from build123d import *

# Parameters (mm, degrees)
F0_W     = 3.6
F0_H     = 1.6955656027
F0_H_2   = 2
F1_DEPTH = 7


with BuildPart() as f1:
    # F0 (on Right) → F1 (new body)
    with BuildSketch(Plane.YZ):
        with Locations((-0.3402145463, -3.3855575087)):
            Rectangle(F0_W, F0_H)
        with Locations((-0.3402145463, -5.2333403101)):
            Rectangle(F0_W, F0_H_2)
        Polygon((-2.1402145463, -6.2333403101), (-2.1402145463, -4.2333403101), (-3.6402145463, -6.2333403101), align=None)
        Polygon((-3.3397897729, -2.5377747074), (-2.1402145463, -2.5377747074), (1.4597854537, -2.5377747074), (2.6593606802, -2.5377747074), (2.6593606802, -0.4877204478), (1.1097854537, -0.4877204478), (-0.3402145463, -0.4877204478), (-1.7902145463, -0.4877204478), (-3.3397897729, -0.4877204478), align=None)
        Polygon((2.9597854537, -6.2333403101), (1.4597854537, -4.2333403101), (1.4597854537, -6.2333403101), align=None)
        Polygon((-3.3402145463, -2.5377747074), (-3.3397897729, -2.5377747074), (-3.3397897729, -0.4877204478), (-4.7602145463, -0.4877204478), (-4.7602145463, 2.0122795522), (-4.508031692, 2.0122795522), (-4.7602145463, 3.5118722885), (-6.076728541, 3.5118722885), (-6.076728541, -2.5377747074), align=None)
        Polygon((2.6593606802, -0.4877204478), (2.6593606802, -2.5377747074), (2.6597854537, -2.5377747074), (5.3962994483, -2.5377747074), (5.3962994483, 3.5118722885), (4.0797854537, 3.5118722885), (3.8276025993, 2.0122795522), (4.0797854537, 2.0122795522), (4.0797854537, -0.4877204478), align=None)
        Polygon((-1.7902145463, 0.3914704144), (-1.7902145463, -0.4877204478), (-0.3402145463, -0.4877204478), (1.1097854537, -0.4877204478), (1.1097854537, 0.3914704144), (-0.3402145463, 0.3914704144), align=None)
    extrude(amount=F1_DEPTH)


solid = f1.part
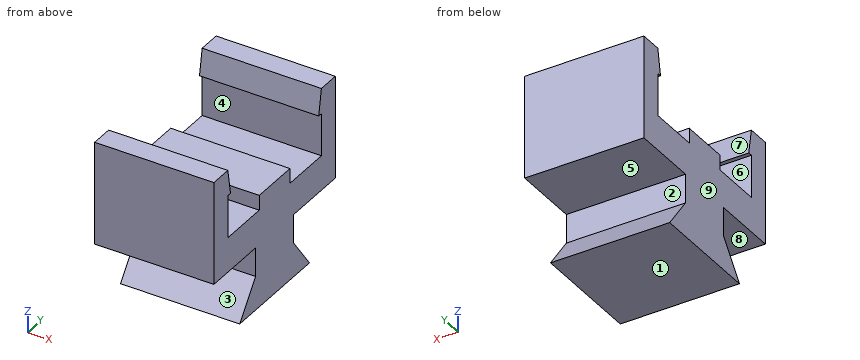
Check sheet for the modelled part. Datum: model origin and axes. Units: mm. Face numbers are marked on the shaded views. A direction names the side the tool comes from. Round coordinates to 2 decimals unless told otherwise and drop trailing zeros. Loops run counter-clockwise (first coordinate to the right, second up) from the corner with the lowest first, then second, coordinate; pieces in that order, holes last.
1. Sectioned sample at B-B on y = 2.5. Record the boundary of the cut face in (x, z).
2. Set-up check for the marked faces 5, 6, 7, 8 and 9: record each of +Z, -Z, +X, -X, +Y, -Y from which the full face is reachable in a straight line by a thin tool's end or side.
3. Mould release check, pull along Y, two halves, no side actions. Record for the marked faces 1, 2, 3 and 4: released by +Y, released by -Y, zero draft, split by the parting line, or undercut.
4. Sectioned sample at C-C on x = 6.75. Record the boundary of the cut face in (y, z), and give its area (3 significant figures).
5. Sectioned sample at D-D on z = -3.25. Record the boundary of the cut face in (x, y).
6. Scan lines: probe 1 along Y at (x, z) = (4.25, 0); probe 2 along Y at (x, z) = (6.25, 1.25); probe 3 along Y at (x, z) = (5.5, -3.5). Record each from-to range of solid material in increasing order.
7. Gauge pin test, flat ends, axial feed: pin 1 Ø1.2 at (x, y) = (4, 4.5) entering from -Z; pin 2 Ø0.5 at (x, z) = (3.5, -3.5) entering from +Y; pin 3 Ø1.5 at (x, y) = (2, 0) entering from +Z. Record the tip position at first contact, or that the pin passes through.
8. Sectioned sample at A-A on z = 2.75. Record the boundary of the cut face in (x, y).
Recorded:
1. outline: (0, -6.23) - (7, -6.23) - (7, -5.62) - (0, -5.62) - close; (0, -2.54) - (7, -2.54) - (7, -0.49) - (0, -0.49) - close
2. face 5: +X, -X, +Y
2. face 6: +X, -X
2. face 7: +Z, +X, -X
2. face 8: +X, -X, -Y
2. face 9: +Z, -Z, -X, +Y, -Y
3. face 1: zero draft
3. face 2: released by +Y
3. face 3: released by -Y
3. face 4: undercut
4. outline: (-6.08, -2.54) - (-2.14, -2.54) - (-2.14, -4.23) - (-3.64, -6.23) - (2.96, -6.23) - (1.46, -4.23) - (1.46, -2.54) - (5.4, -2.54) - (5.4, 3.51) - (4.08, 3.51) - (3.83, 2.01) - (4.08, 2.01) - (4.08, -0.49) - (1.11, -0.49) - (1.11, 0.39) - (-1.79, 0.39) - (-1.79, -0.49) - (-4.76, -0.49) - (-4.76, 2.01) - (-4.51, 2.01) - (-4.76, 3.51) - (-6.08, 3.51) - close
4. area: 53.3 mm2
5. outline: (0, -2.14) - (7, -2.14) - (7, 1.46) - (0, 1.46) - close
6. probe 1: y = -6.08 to -4.76, -1.79 to 1.11, 4.08 to 5.4
6. probe 2: y = -6.08 to -4.76, 4.08 to 5.4
6. probe 3: y = -2.14 to 1.46
7. pin 1: stops at z = -2.54
7. pin 2: stops at y = 1.46
7. pin 3: stops at z = 0.39
8. outline: (0, -6.08) - (7, -6.08) - (7, -4.63) - (0, -4.63) - close; (0, 3.95) - (7, 3.95) - (7, 5.4) - (0, 5.4) - close
